from build123d import *

# Parameters (mm, degrees)
F0_W      = 40.64
F0_H      = 77.47
F1_DEPTH  = 1.5
F2_W      = 40.64
F2_H      = 8.382
F3_DEPTH  = 10.16
F4_W      = 10.16
F4_H      = 8.382
F5_DEPTH  = 10.16
F7_DEPTH  = 1.5
F9_DEPTH  = 12.7
F10_W     = 7.62
F10_H     = 9.271
F11_DEPTH = 3.81


with BuildPart() as f1:
    # F0 (on Top) → F1 (new body)
    with BuildSketch(Plane.XY):
        Rectangle(F0_W, F0_H)
    extrude(amount=F1_DEPTH)

    # F2 (on face) → F3 (join)
    with BuildSketch(Plane.XY.offset(1.5)):
        with Locations((0, 34.544)):
            Rectangle(F2_W, F2_H)
        with Locations((0, -34.544)):
            Rectangle(F2_W, F2_H)
    extrude(amount=F3_DEPTH)

    # F4 (on face) → F5 (cut, through all)
    with BuildSketch(Plane.XY.offset(11.66)):
        with Locations((-15.24, 34.544)):
            Rectangle(F4_W, F4_H)
        with Locations((15.24, 34.544)):
            Rectangle(F4_W, F4_H)
    extrude(amount=-F5_DEPTH, mode=Mode.SUBTRACT)

    # F6 (on face) → F7 (cut, through all)
    with BuildSketch(Plane.XY.offset(1.5)):
        with BuildLine():
            ThreePointArc((-15.24, 31.115), (-13.4439487758, 31.8589487758), (-12.7, 33.655))
            ThreePointArc((-12.7, 33.655), (-13.4439487758, 35.4510512242), (-15.24, 36.195))
            ThreePointArc((-15.24, 36.195), (-17.0360512242, 35.4510512242), (-17.78, 33.655))
            ThreePointArc((-17.78, 33.655), (-17.0360512242, 31.8589487758), (-15.24, 31.115))
        make_face()
        with BuildLine():
            ThreePointArc((15.24, 36.195), (13.4439487758, 35.4510512242), (12.7, 33.655))
            ThreePointArc((12.7, 33.655), (13.4439487758, 31.8589487758), (15.24, 31.115))
            ThreePointArc((15.24, 31.115), (17.0360512242, 31.8589487758), (17.78, 33.655))
            ThreePointArc((17.78, 33.655), (17.0360512242, 35.4510512242), (15.24, 36.195))
        make_face()
        with BuildLine():
            ThreePointArc((17.78, -26.035), (17.0360512242, -24.2389487758), (15.24, -23.495))
            ThreePointArc((15.24, -23.495), (13.4439487758, -24.2389487758), (12.7, -26.035))
            ThreePointArc((12.7, -26.035), (15.24, -28.575), (17.78, -26.035))
        make_face()
        with BuildLine():
            ThreePointArc((-15.24, -23.495), (-17.0360512242, -27.8310512242), (-12.7, -26.035))
            ThreePointArc((-12.7, -26.035), (-13.4439487758, -24.2389487758), (-15.24, -23.495))
        make_face()
    extrude(amount=-F7_DEPTH, mode=Mode.SUBTRACT)

    # F8 (on face) → F9 (join)
    with BuildSketch(Plane.XY.offset(1.5)):
        Polygon((8.89, -26.797), (8.89, 16.383), (0, 16.383), (-8.89, 16.383), (-8.89, -26.797), align=None)
    extrude(amount=F9_DEPTH)

    # F10 (on face) → F11 (join)
    with BuildSketch(Plane.XY.offset(14.2)):
        with Locations((0, -22.1615)):
            Rectangle(F10_W, F10_H)
    extrude(amount=F11_DEPTH)


solid = f1.part
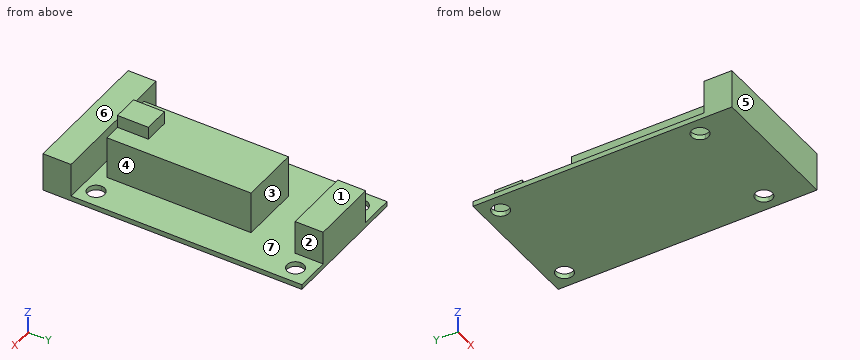
Verification items for the finished model (mm, model axes). Face numbers are marked on the shaded views. A direction names the side the tool comes from. Coordinates: 2 decimals unless noted, no trailing zeros. Order: outer loops, then holes, each group sorted by start corner. A loop starts at its lowest first (then second) coordinate and runs counter-clockwise, first axis right, second up. Notation, with made-up numbers: M 59,12 L 103,12 A25 cw 103,51 Z; hole C 19.25,9 d3. An arc over 180 degrees is marked long. Return JSON: item names as keys, results as strings.
1) Cross-section at A-A, the plane x = -6. Record the boundary of the cut face in (y, z) (3 decimals), and give its area (3 significant figures).
Answer list:
{"outline": "M -38.735,0 L 38.735,0 L 38.735,11.66 L 30.353,11.66 L 30.353,1.5 L 16.383,1.5 L 16.383,14.2 L -26.797,14.2 L -26.797,1.5 L -30.353,1.5 L -30.353,11.66 L -38.735,11.66 Z", "area": "835 mm2"}
2) Cross-section at B-B, the plane y = -4.5. Record the boundary of the cut face in (x, z), and give its area (3 significant figures).
Answer list:
{"outline": "M -20.32,0 L 20.32,0 L 20.32,1.5 L 8.89,1.5 L 8.89,14.2 L -8.89,14.2 L -8.89,1.5 L -20.32,1.5 Z", "area": "287 mm2"}
3) Cross-section at D-D, the plane x = 11.5. Record the boundary of the cut face in (y, z) (3 decimals).
Answer list:
{"outline": "M -38.735,0 L 38.735,0 L 38.735,1.5 L -30.353,1.5 L -30.353,11.66 L -38.735,11.66 Z"}
4) Access from +Z, -Z, +X, -X, +Y, -Y to the whole of each face (thin tool, end or side, straight path). Record for the marked faces 1, 2 and 3.
Answer list:
{"face 1": "+Z, +X, -X, +Y", "face 2": "+Z, +X, +Y", "face 3": "+Z, +X, -X"}
5) Release check for a two-part mould opening along Y. For the marked faces 4, 5, 6 and 7 record: +Y half, -Y half, draft (parallel to the pull), parting line (faces both ways), or undercut.
Answer list:
{"face 4": "undercut", "face 5": "-Y half", "face 6": "draft", "face 7": "undercut"}
6) Cross-section at C-C, the plane x = -16. Record the boundary of the cut face in (y, z) (3 decimals), and give its area (3 significant figures).
Answer list:
{"outline": "M -38.735,0 L -28.459,0 L -28.459,1.5 L -30.353,1.5 L -30.353,11.66 L -38.735,11.66 Z; M -23.611,0 L 31.231,0 L 31.231,1.5 L -23.611,1.5 Z; M 36.079,0 L 38.735,0 L 38.735,1.5 L 36.079,1.5 Z", "area": "187 mm2"}
7) Gauge pin test, flat ends, axial feed: pin 1 (6 mm diameter, centred on x = -15.24, y = -26.035, fed in from +Z); pin 2 (3 mm diameter, centred on y = -20.5, z = 17, fed in from +X); pin 3 (9 mm diameter, centred on y = 33, z = 7, fed in from -X). Record the tip position at first contact, or that the pin passes through.
Answer list:
{"pin 1": "z = 1.5", "pin 2": "x = 3.81", "pin 3": "x = -10.16"}
8) Thickness scan on L1, parallel to Y at x = 0.5, z = 10.5 (3 decimals); L2, parallel to Y at x = -15.24, z = 0.85 (3 decimals); L3, parallel to Z at x = -12, y = -24.5. Record the ranges inside material, lowest first. Write a range as [from, to].
Answer list:
{"L1": "[-38.735, -30.353], [-26.797, 16.383], [30.353, 38.735]", "L2": "[-38.735, -28.575], [-23.495, 31.115], [36.195, 38.735]", "L3": "[0, 1.5]"}
